```python
from build123d import *

# Parameters (mm, degrees)
Y_KSEKLIK_EKSTR_ZYON1_DEPTH = 54
IZIM2_R                     = 5
Y_KSEKLIK_EKSTR_ZYON2_DEPTH = 8
FEDER2_REACH                = 82.985
IZIM6_WALL_W                = 203.630625642
IZIM6_WALL_H                = 6
Y_KSEKLIK_EKSTR_ZYON3_START = 8
IZIM7_R                     = 14
IZIM7_R_2                   = 5
Y_KSEKLIK_EKSTR_ZYON3_DEPTH = 8
RADYUS1_R                   = 10
RADYUS2_START               = 13.0000001
RADYUS2_DEPTH               = 27.9999998
RADYUS2_2_DEPTH             = 54
RADYUS2_START_2             = -1.083333333
RADYUS2_3_DEPTH             = 8
RADYUS3_R                   = 10
IZIM9_R                     = 2.5
KES_EKSTR_ZYON1_DEPTH       = 87.763127471


with BuildPart() as part:
    # Çizim1 → Yükseklik-Ekstrüzyon1 (new body)
    with BuildSketch(Plane(origin=(0, 0, 0), x_dir=(0, 0, -1), z_dir=(1, 0, 0))):
        Polygon((-6.916666667, 9.833333333), (-36.916666667, 9.833333333), (-36.916666667, 1.833333333), (-19.333333333, 1.833333333), (1.083333333, 1.833333333), (1.083333333, 5.833333333), (-6.916666667, 5.833333333), align=None)
    extrude(amount=Y_KSEKLIK_EKSTR_ZYON1_DEPTH)

    # Çizim2 → Yükseklik-Ekstrüzyon2 (add)
    with BuildSketch(Plane(origin=(0, 0, 6.916666667), x_dir=(-1, 0, 0), z_dir=(0, 0, -1))):
        with BuildLine():
            ThreePointArc((-13, 52.833333333), (-27, 66.833333333), (-41, 52.833333333))
            Line((-41, 52.833333333), (-41, 9.833333333))
            Line((-41, 9.833333333), (-13, 9.833333333))
            Line((-13, 9.833333333), (-13, 52.833333333))
        make_face()
        with Locations((-27, 52.833333333)):
            Circle(IZIM2_R, mode=Mode.SUBTRACT)
    extrude(amount=-Y_KSEKLIK_EKSTR_ZYON2_DEPTH)

    # Çizim6 wall → Feder2 (add, up to next)
    with BuildSketch(Plane(origin=(27, 26.333333333, 25.916666667), x_dir=(0, 0.832050294338, -0.554700196225), z_dir=(0, 0.554700196225, 0.832050294338)), mode=Mode.PRIVATE) as feder2_sk1:
        Rectangle(IZIM6_WALL_W, IZIM6_WALL_H)
    feder2_tool1 = extrude(feder2_sk1.sketch, amount=-FEDER2_REACH, mode=Mode.PRIVATE) - part.part
    add(feder2_tool1.solids().sort_by_distance((27, 26.333333333, 25.916666667))[0])

    # Çizim7 → Yükseklik-Ekstrüzyon3 (add)
    with BuildSketch(Plane(origin=(0, 0, 6.916666667), x_dir=(-1, 0, 0), z_dir=(0, 0, -1)).offset(Y_KSEKLIK_EKSTR_ZYON3_START)):
        with Locations((-27, 52.833333333)):
            Circle(IZIM7_R)
        with Locations((-27, 52.833333333)):
            Circle(IZIM7_R_2, mode=Mode.SUBTRACT)
    extrude(amount=-Y_KSEKLIK_EKSTR_ZYON3_DEPTH)

    # Radyus1
    radyus1_edges = [part.edges().sort_by_distance(p)[0] for p in [
        (13, 9.833333333, 10.916666667),
        (41, 9.833333333, 10.916666667),
    ]]
    fillet(radyus1_edges, radius=RADYUS1_R)

    # Radyus2: read off the stored shape, not the designer's step
    # Radyus2 outline → Radyus2 (add)
    with BuildSketch(Plane.YZ.offset(RADYUS2_START)):
        with BuildLine():
            Line((5.833333333, 6.916666667), (5.833333333, -1.083333333))
            ThreePointArc((5.833333333, -1.083333333), (9.306736984, 4.662633359), (15.631292304, 6.916666667))
            Line((15.631292304, 6.916666667), (5.833333333, 6.916666667))
        make_face()
    extrude(amount=RADYUS2_DEPTH)

    # Radyus2 2 outline → Radyus2 2 (add)
    with BuildSketch(Plane.YZ):
        with BuildLine():
            Line((5.833333333, 6.916666667), (5.833333333, -1.083333333))
            ThreePointArc((5.833333333, -1.083333333), (9.306736984, 4.662633359), (15.631292304, 6.916666667))
            Line((15.631292304, 6.916666667), (5.833333333, 6.916666667))
        make_face()
    extrude(amount=RADYUS2_2_DEPTH)

    # Radyus2 3 outline → Radyus2 3 (cut)
    with BuildSketch(Plane.XY.offset(RADYUS2_START_2)):
        with BuildLine():
            Line((-1, 9.833333333), (3, 9.833333333))
            ThreePointArc((3, 9.833333333), (8.986094999, 11.822923439), (12.590214921, 17))
            Line((12.590214921, 17), (-1, 17))
            Line((-1, 17), (-1, 9.833333333))
        make_face()
        with BuildLine():
            Line((55, 17), (41.409785079, 17))
            ThreePointArc((41.409785079, 17), (45.013905001, 11.822923439), (51, 9.833333333))
            Line((51, 9.833333333), (55, 9.833333333))
            Line((55, 9.833333333), (55, 17))
        make_face()
    extrude(amount=RADYUS2_3_DEPTH, mode=Mode.SUBTRACT)

    # Radyus3
    radyus3_edges = [part.edges().sort_by_distance(p)[0] for p in [
        (54, 5.833333333, 36.916666667),
        (0, 5.833333333, 36.916666667),
    ]]
    fillet(radyus3_edges, radius=RADYUS3_R)

    # Çizim9 → Kes-Ekstrüzyon1 (cut, through all)
    with BuildSketch(Plane(origin=(0, 9.833333333, 0), x_dir=(1, 0, 0), z_dir=(0, 1, 0))):
        with Locations(Location((9, -26.916666667, 0), (0, 0, 270))):
            Circle(IZIM9_R)
        with Locations(Location((45, -26.916666667, 0), (0, 0, 270))):
            Circle(IZIM9_R)
    extrude(amount=-KES_EKSTR_ZYON1_DEPTH, mode=Mode.SUBTRACT)


solid = part.part
```
Read the model definition and answer for the solid it produces. Units are mm, in the model's axes. A direction names the side the tool comes from. Coordinates: 2 decimals unless noted, no trailing zeros. Write each loop counter-clockwise with the first axis right and the second up, starting at its lowest first coordinate (ties: lowest second). Pieces come first, ordered by that corner, then holes. Notation, with made-up numbers: (-26, 85.5) - (31, 85.5) arc R17 ccw to (31, 104.5) - close; hole circle Ø9 at (89.5, 62.25). An arc over 180 degrees is marked (long way). Answer as a JSON object with one key per item and string values. Group by question number.
1. A cutting plane is placed at B-B (z = 9). Determine the outline of the cut face in (x, y), plus the area to 3 significant figures.
2. Consider L1, parallel to Y at x = 27, z = 2.5; L2, parallel to Y at x = 27, z = 6; L3, parallel to Y at x = 2.5, z = 6.5. Determine where each line is inside the solid, lowest interval first. Write a range as [from, to].
3. The mould has two halves that part along Z. Classify faces 6 (the flat face through (27, 47, -1.083)), 7 (the flat face through (27, 6, 36.917)), 8 (the cylindrical face through (42.56, 5.89, 26.37)): +Z half, -Z half, draft (parallel to the pull), parting line (faces both ways), or undercut.
4. Each of these flat-tipped pins is pushed along its axis until it touches: P1, Ø11, axis at y = 28.5, z = 29.5, coming from the -X side; P2, Ø1.5, axis at x = 21, z = 9.5, coming from the +Y side; P3, Ø6, axis at y = 17.5, z = 29.5, coming from the +X side. Where does it stop, or does it pass through?
5. A cutting plane is placed at C-C (y = 8). Determine the outline of the cut face in (x, z).
6. A cutting plane is placed at A-A (x = 27). Determine the outline of the cut face in (y, z).
7. Which of the six approach directions +Z, -Z, +X, -X, +Y, -Y give full straight-line access (tool end or side, diameter ignored) to faces 1 (the flat face through (33, 39, 14.917)), 2 (the cylindrical face through (26.62, 8.14, 3.54)), 3 (the flat face through (30, 22, 20)), 4 (the flat face through (13, 36, 11)), 5 (the flat face through (41, 37, 11))?
8. A cutting plane is placed at D-D (x = 4). Determine the outline of the cut face in (y, z), plus the area to 3 significant figures.
Worked out:
{
 "1": {"outline": "(0, 1.83) - (54, 1.83) - (54, 9.83) - (51, 9.83) arc R10 cw to (41, 19.83) - (41, 52.83) arc R14 ccw to (13, 52.83) - (13, 19.83) arc R10 cw to (3, 9.83) - (0, 9.83) - close; hole circle Ø10 at (27, 52.83)", "area": "1,910 mm²"},
 "2": {"L1": "y = [1.83, 7.34], [38.83, 47.83], [57.83, 66.83]", "L2": "y = [1.83, 11.45], [38.83, 47.83], [57.83, 66.83]", "L3": "y = [1.83, 9.83]"},
 "3": {"face 6": "-Z half", "face 7": "+Z half", "face 8": "undercut"},
 "4": {"P1": "stops at x = 24", "P2": "stops at y = 65.81", "P3": "stops at x = 30"},
 "5": {"outline": "(0, 3.38) - (54, 3.38) - (54, 26.92) arc R10 ccw to (44, 36.92) - (10, 36.92) arc R10 ccw to (0, 26.92) - close; hole circle Ø5 at (9, 26.92); hole circle Ø5 at (45, 26.92)"},
 "6": {"outline": "(1.83, -1.08) - (5.83, -1.08) arc R10 cw to (15.63, 6.92) - (38.83, 6.92) - (38.83, -1.08) - (47.83, -1.08) - (47.83, 14.92) - (42.83, 14.92) - (9.83, 36.92) - (1.83, 36.92) - close; (57.83, -1.08) - (66.83, -1.08) - (66.83, 14.92) - (57.83, 14.92) - close"},
 "7": {"face 1": "+Z, +Y", "face 2": "-Z, +X, -X", "face 3": "+Z, +X, +Y", "face 4": "+Z, -Z, -X, +Y", "face 5": "+Z, -Z, +X, +Y"},
 "8": {"outline": "(1.83, -1.08) - (5.83, -1.08) arc R10 cw to (9.88, 5.1) - (9.88, 14.92) - (9.83, 14.92) - (9.83, 34.92) - (1.83, 34.92) - close", "area": "273 mm²"}
}
